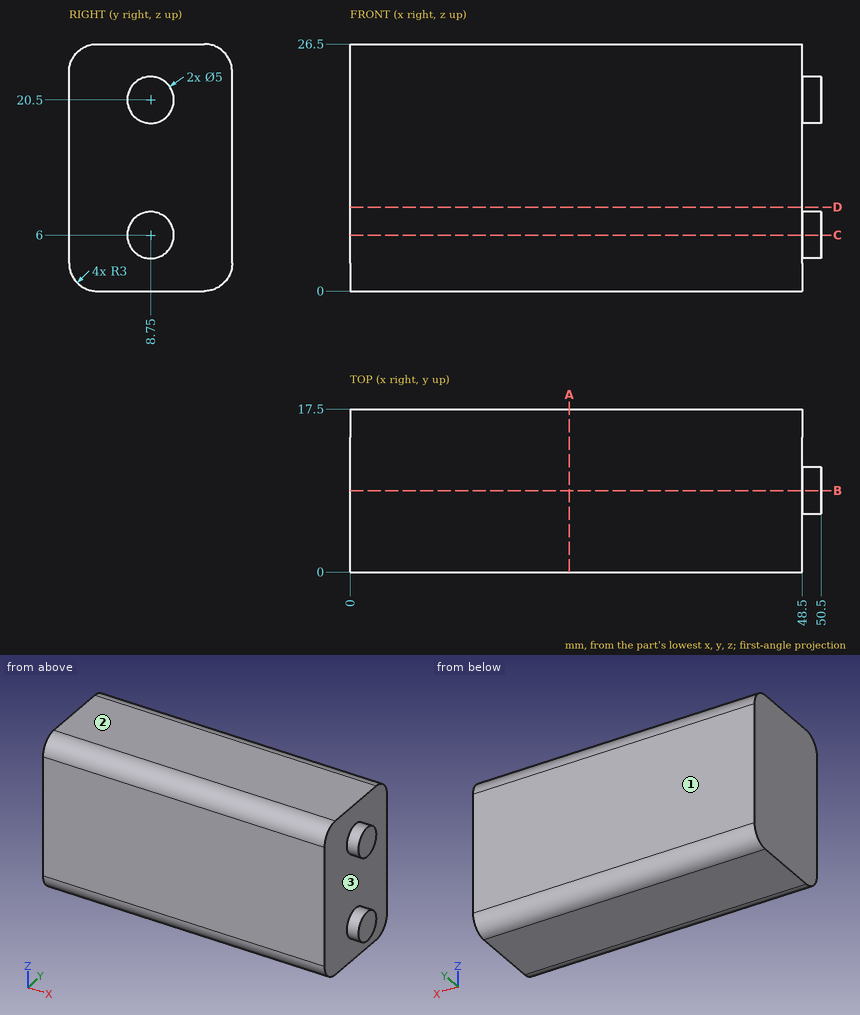
Study the drawing (mm; zero at the part's minimum x, y, z) and answer. Give positions to 0.01 mm unless a question says otherwise; leave off trailing zeros. Write each loop counter-clockwise with the first axis right and the second up, starting at its lowest first coordinate (ties: lowest second). Pieces come first, ordered by that corner, then holes. Notation, with made-up numbers: (-35, 47.5) -> (5, 47.5) arc R29 ccw to (5, 78.5) -> close; hole circle Ø2 at (48.5, 8.5). An arc over 180 degrees is marked (long way). Write item = value, one per line. Start each with the question number.
1) The part is cut by section D-D, the plane z = 9. Determine the outline of the cut face in (x, y), and give its area (3 significant figures).
2) Straight lines are drawn through the part: line 1 along X through (y, z) = (10.25, 18.25); line 2 along Y through (x, z) = (32.5, 23.75); line 3 along Z through (x, y) = (8, 1.25). For each, find the intervals that lie inside material, in ascending order.
3) The part is cut by section B-B, the plane y = 8.75. Determine the outline of the cut face in (x, z).
4) The part is cut by section C-C, the plane z = 6. Determine the outline of the cut face in (x, y), and give its area (3 significant figures).
5) The part is cut by section A-A, the plane x = 23.5. Determine the outline of the cut face in (y, z), and give its area (3 significant figures).
6) Determine the mould class of the marked faces 1, 2 and 3 for opening direction Z: +Z half, -Z half, draft (parallel to the pull), parting line (faces both ways), or undercut.
7) This flat-tipped pin is pushed along its axis until it touches: pin 1 (2 mm diameter, centred on x = 10, z = 17, fed in from -Y). Where does it stop, or does it pass through?
Solutions:
q1.outline = (0, 0) -> (48.5, 0) -> (48.5, 17.5) -> (0, 17.5) -> close
q1.area = 849 mm²
q2.line_1 = 0 to 48.5
q2.line_2 = 0.01 to 17.49
q2.line_3 = 0.56 to 25.94
q3.outline = (0, 0) -> (48.5, 0) -> (48.5, 3.5) -> (50.5, 3.5) -> (50.5, 8.5) -> (48.5, 8.5) -> (48.5, 18) -> (50.5, 18) -> (50.5, 23) -> (48.5, 23) -> (48.5, 26.5) -> (0, 26.5) -> close
q4.outline = (0, 0) -> (48.5, 0) -> (48.5, 6.25) -> (50.5, 6.25) -> (50.5, 11.25) -> (48.5, 11.25) -> (48.5, 17.5) -> (0, 17.5) -> close
q4.area = 859 mm²
q5.outline = (0, 3) arc R3 ccw to (3, 0) -> (14.5, 0) arc R3 ccw to (17.5, 3) -> (17.5, 23.5) arc R3 ccw to (14.5, 26.5) -> (3, 26.5) arc R3 ccw to (0, 23.5) -> close
q5.area = 456 mm²
q6.face_1 = draft
q6.face_2 = +Z half
q6.face_3 = undercut
q7.pin_1 = 0
